```python
from build123d import *
from build123d.topology import SkipClean

# Parameters (mm, degrees)
SKETCH3_R                = 100
BOSS_EXTRUDE1_DEPTH      = 90
BOSS_EXTRUDE2_REACH      = 285.901
BOSS_EXTRUDE2_END_RADIUS = 100
SKETCH4_R                = 45
SKETCH5_R                = 40
BOSS_EXTRUDE3_DEPTH      = 5


with BuildPart() as part:
    # Sketch3 → Boss-Extrude1 (new body)
    with BuildSketch(Plane(origin=(0, 0, 0), x_dir=(0, 0, -1), z_dir=(1, 0, 0))):
        with Locations(Location((0, 0, 0), (0, 0, 180))):
            Circle(SKETCH3_R)
    extrude(amount=BOSS_EXTRUDE1_DEPTH)

    # Boss-Extrude2: up to this cylinder (the profile starts outside it)
    with SkipClean():  # the faces are left unmerged after this step: merging them gives an invalid solid
        boss_extrude2_end = Plane(origin=(45, 0, 0), z_dir=(-1, 0, 0)) * Cylinder(BOSS_EXTRUDE2_END_RADIUS, 772.802, mode=Mode.PRIVATE)
        # Sketch4 → Boss-Extrude2 (add, up to the surface)
        with BuildSketch(Plane(origin=(0, 150, 0), x_dir=(1, 0, 0), z_dir=(0, 1, 0)), mode=Mode.PRIVATE) as boss_extrude2_sk1:
            with Locations(Location((45, 0, 0), (0, 0, 270))):
                Circle(SKETCH4_R)
        boss_extrude2_tool1 = extrude(boss_extrude2_sk1.sketch, amount=-BOSS_EXTRUDE2_REACH, mode=Mode.PRIVATE) - boss_extrude2_end
        add(boss_extrude2_tool1.solids().sort_by_distance((45, 150, 0))[0])

    # Sketch5 → Boss-Extrude3 (add)
    with SkipClean():  # the faces are left unmerged after this step: merging them gives an invalid solid
        with BuildSketch(Plane(origin=(0, 150, 0), x_dir=(1, 0, 0), z_dir=(0, 1, 0))):
            with Locations(Location((45, 0, 0), (0, 0, 270))):
                Circle(SKETCH5_R)
        extrude(amount=BOSS_EXTRUDE3_DEPTH)


solid = part.part
```
Can you work these out from the model? Positions are in its coordinate system, mm. A direction names the side the tool comes from. Give positions to 0.01 mm unless a question says otherwise; leave off trailing zeros. Order: outer loops, then holes, each group sorted by start corner. A loop starts at its lowest first (then second) coordinate and runs counter-clockwise, first axis right, second up. Notation, with made-up numbers: (-7.5, 15.5) - (47.5, 15.5) arc R27 ccw to (47.5, 48.5) - close; hole circle Ø9 at (-9, 87.5). An arc over 180 degrees is marked (long way). Use a Markdown table: item, result. Add a question column.
Q1. If we section it at C-C on y = 125.5: Write out the boundary of the cut face in (x, z), plus the area to 3 significant figures.
Q2. If we section it at B-B on z = -28: Write out the boundary of the cut face in (x, y).
Q3. On a 3-axis mill with a long thin cutter (end or side, diameter ignored), from which of +Z, -Z, +X, -X, +Y, -Y can I reach the whole of each face in a straight line? I mean faces 1 (the flat face through (0, -1, -1)), 2 (the cylindrical face through (27.765, 120.076, 41.569)). Say none if no direction works.
Q4. I'm going to push flat-ended pins straight in: pin 1 (4 mm diameter, centred on x = 20.5, y = 23, fed in from -Z); pin 2 (1 mm diameter, centred on x = 52.5, z = 74.5, fed in from +Y); pin 3 (1 mm diameter, centred on x = 66, y = 97, fed in from -Z). Where does each tip first touch, or does it pass through?
Q5. If we section it at D-D on x = 19: Write out the boundary of the cut face in (y, z), plus the area to 3 significant figures.
Q6. If we section it at A-A on x = 81: Write out the boundary of the cut face in (y, z).
Q7. Please list where these lines run through material, in increasing order: line 1 along Y through (x, z) = (66, 2); line 2 along Z through (x, y) = (44.5, 101); line 3 along Z through (x, y) = (53, 77).
Answers follow:
| question | item | result |
|---|---|---|
| 1 | outline | circle Ø90 at (45, 0) |
| 1 | area | 6,360 mm^2 |
| 2 | outline | (0, -96) - (90, -96) - (90, 96) - (80.23, 96) - (80.23, 150) - (73.57, 150) - (73.57, 155) - (16.43, 155) - (16.43, 150) - (9.77, 150) - (9.77, 96) - (0, 96) - close |
| 3 | face 1 | +Z, -Z, -X, +Y, -Y |
| 3 | face 2 | +Y |
| 4 | pin 1 | stops at z = -97.77 |
| 4 | pin 2 | stops at y = 67.26 |
| 4 | pin 3 | stops at z = -40.06 |
| 5 | outline | (93.01, -36.73) - (150, -36.73) - (150, -30.4) - (155, -30.4) - (155, 30.4) - (150, 30.4) - (150, 36.73) - (93.01, 36.73) arc R100 ccw (long way) to start |
| 5 | area | 35,600 mm^2 |
| 6 | outline | (96.29, -27) - (150, -27) - (150, -17.44) - (155, -17.44) - (155, 17.44) - (150, 17.44) - (150, 27) - (96.29, 27) arc R100 ccw (long way) to start |
| 7 | line 1 | y = -99.98 to 155 |
| 7 | line 2 | z = -45 to 45 |
| 7 | line 3 | z = -63.8 to 63.8 |
